Could you check a few things on this model? Use its own coordinates, in mm. A direction names the side the tool comes from. Coordinates: 2 decimals unless noted, no trailing zeros. Order: outer loops, then holes, each group sorted by start corner. A loop starts at its lowest first (then second) coordinate and runs counter-clockwise, first axis right, second up. Notation, with made-up numbers: (62, 78.5) - (98, 78.5) arc R20 ccw to (98, 114.5) - close; hole circle Ø8 at (-18, 86.5). An arc over 180 degrees is marked (long way). One line per item, written item: value.
from build123d import *

# Parameters (mm, degrees)
F0_W     = 6.35
F0_H     = 6.35
F0_R     = 1.1751262937
F1_DEPTH = 6.35
F2_DEPTH = 3.175


# Not quite as in the source:
# - a feature names something its author has since deleted; it is built from what else it names


with BuildPart() as f1:
    # F0 (on Top) → F1 (new body)
    with BuildSketch(Plane.XY):
        with Locations((3.175, 3.175)):
            Rectangle(F0_W, F0_H)
        with Locations((3.175, 3.175)):
            Circle(F0_R, mode=Mode.SUBTRACT)
    extrude(amount=F1_DEPTH)



with BuildPart() as f1b:
    # F0 (on Top) → F1, piece 2 (new body)
    with BuildSketch(Plane.XY):
        with Locations((15.875, 3.175)):
            Rectangle(F0_W, F0_H)
    extrude(amount=F1_DEPTH)


with BuildPart() as f1_1:
    add(f1.part)

    add(f1b.part)  # F2 merges F1b
    # F0 (on Top) → F2 (join)
    with BuildSketch(Plane.XY):
        with Locations((9.525, 3.175)):
            Rectangle(F0_W, F0_H)
    extrude(amount=F2_DEPTH)


solid = f1_1.part
Item 1: For faces 5 (the face through (5, 3, 6.35)), 6 (the face through (12.7, 3, 5)), which set-ups out of +Z, -Z, +X, -X, +Y, -Y let a thin tool reach every point of the face, with its end or its side?
Conclusion:
face 5: +Z, +X, -X, +Y, -Y
face 6: +Z, +Y, -Y
Item 2: I want a section at B-B on y = 5. Please give me the cut outline in (x, z) (3 decimals).
Conclusion:
outline: (0, 0) - (19.05, 0) - (19.05, 6.35) - (12.7, 6.35) - (12.7, 3.175) - (6.35, 3.175) - (6.35, 6.35) - (0, 6.35) - close
Item 3: I want a section at D-D on z = 2.5. Please give me the cut outline in (x, y) (3 decimals), then the cut area to 3 significant figures.
Conclusion:
outline: (0, 0) - (19.05, 0) - (19.05, 6.35) - (0, 6.35) - close; hole circle Ø2.35 at (3.175, 3.175)
area: 117 mm²
Item 4: I want a section at A-A on z = 4.75. Please give me the cut outline in (x, y) (3 decimals), then the cut area to 3 significant figures.
Conclusion:
outline: (0, 0) - (6.35, 0) - (6.35, 6.35) - (0, 6.35) - close; (12.7, 0) - (19.05, 0) - (19.05, 6.35) - (12.7, 6.35) - close; hole circle Ø2.35 at (3.175, 3.175)
area: 76.3 mm²
Item 5: If I drill on probe 1 along Y at (x, z) = (3.25, 6.25); probe 2 along X at (y, z) = (4.75, 4.5); probe 3 along X at (y, z) = (3, 5), over which ranges is the centre line in solid material (lowest first)?
Conclusion:
probe 1: 0 to 2, 4.35 to 6.35
probe 2: 0 to 6.35, 12.7 to 19.05
probe 3: 0 to 2.01, 4.34 to 6.35, 12.7 to 19.05
Item 6: I'm going to push flat-ended pins straight in: pin 1 Ø1.9 at (x, y) = (8.5, 2.5) entering from +Z (3 decimals); pin 2 Ø1.9 at (x, y) = (3.175, 3.175) entering from +Z. Where does each tip first touch, or does it pass through?
Conclusion:
pin 1: z = 3.175
pin 2: through
Item 7: I want a section at C-C on x = 2.5. Please give me the cut outline in (y, z), then the cut area to 3 significant figures.
Conclusion:
outline: (0, 0) - (2.21, 0) - (2.21, 6.35) - (0, 6.35) - close; (4.14, 0) - (6.35, 0) - (6.35, 6.35) - (4.14, 6.35) - close
area: 28.1 mm²
Item 8: Thinking about a two-plate mould opening in Y: for faces 1 (the face through (9, 6.35, 3)), 2 (the face through (6.35, 3, 5)), 3 (the face through (4.296, 3.528, 3.131)), 4 (the face through (9, 0, 3)), which applies, pulls with the +Y half, pulls with the -Y half, needs draft (parallel to the pull), parting line crosses it, or undercut?
Conclusion:
face 1: pulls with the +Y half
face 2: needs draft
face 3: undercut
face 4: pulls with the -Y half
